```python
from build123d import *

# Parameters (mm, degrees)
F0_W     = 40
F0_H     = 3
F1_DEPTH = 12.5
F2_DEPTH = 9.5
F0_R     = 3.73
F3_DEPTH = 9.5
F4_DEPTH = 1.5
F5_W     = 13
F5_H     = 3
F6_DEPTH = 40


with BuildPart() as f1:
    # F0 (on Right) → F1 (new body, symmetric)
    with BuildSketch(Plane.YZ):
        with Locations((20, 1.5)):
            Rectangle(F0_W, F0_H)
    extrude(amount=F1_DEPTH, both=True)

    # F0 (on Right) → F2 (join, symmetric)
    with BuildSketch(Plane.YZ):
        Polygon((0, 7), (0, 3), (40, 3), (40, 7), (28.54, 7), align=None)
    extrude(amount=F2_DEPTH, both=True)

    # F0 (on Right) → F3 (join, symmetric)
    with BuildSketch(Plane.YZ):
        with BuildLine():
            Line((28.54, 7), (40, 7))
            Line((40, 7), (40, 18.87))
            ThreePointArc((40, 18.87), (37.212814, 23.786579), (31.562741, 23.920114))
            ThreePointArc((31.562741, 23.920114), (29.353421, 21.812814), (28.54, 18.87))
            Line((28.54, 18.87), (28.54, 7))
        make_face()
        with Locations((34.27, 18.87)):
            Circle(F0_R, mode=Mode.SUBTRACT)
    extrude(amount=F3_DEPTH, both=True)

    # F0 (on Right) → F4 (join, symmetric)
    with BuildSketch(Plane.YZ):
        with BuildLine():
            Line((31.562741, 23.920114), (0, 7))
            Line((0, 7), (28.54, 7))
            Line((28.54, 7), (28.54, 18.87))
            ThreePointArc((28.54, 18.87), (29.353421, 21.812814), (31.562741, 23.920114))
        make_face()
    extrude(amount=F4_DEPTH, both=True)

    # F5 (on face) → F6 (cut, through all)
    with BuildSketch(Plane.XZ):
        with Locations((0, 1.5)):
            Rectangle(F5_W, F5_H)
    extrude(amount=-F6_DEPTH, mode=Mode.SUBTRACT)


solid = f1.part
```
Check sheet for the modelled part. Datum: model origin and axes. Units: mm. A direction names the side the tool comes from. Round coordinates to 2 decimals unless told otherwise and drop trailing zeros. Loops run counter-clockwise (first coordinate to the right, second up) from the corner with the lowest first, then second, coordinate; pieces in that order, holes last. Notation, with made-up numbers: (46.25, 9.25) - (56.25, 9.25) arc R11 cw to (56.25, 28.25) - close; hole circle Ø11 at (32.25, -14.75). An arc over 180 degrees is marked (long way). Write item = value, one per line. Start each with the question number.
Q1. Section check D-D (y = 12.5). Record the boundary of the cut face in (x, z).
Q2. Section check C-C (z = 19.75). Record the boundary of the cut face in (x, y), plus the area to 3 significant figures.
Q3. Thickness scan on L1, parallel to Z at x = -4, y = 34.27; L2, parallel to X at y = 27.5, z = 2; L3, parallel to X at y = 13, z = 5.75. Record the ranges inside material, lowest first.
Q4. Section check A-A (y = 34.27). Record the boundary of the cut face in (x, z).
Q5. Access from +Z, -Z, +X, -X, +Y, -Y to the whole of each face (thin tool, end or side, straight path). Record for faces 1 (the face through (11, 20, 3)), 2 (the face through (6, 14, 7)), 3 (the face through (0, 20, 3)).
Q6. Release check for a two-part mould opening along X. For faces 4 (the face through (-9.5, 29, 9)), 5 (the face through (-5, 14, 7)), 6 (the face through (-6.5, 20, 1)) record: pulls with the +X half, pulls with the -X half, needs draft (parallel to the pull), parting line crosses it, or undercut.
Q7. Section check B-B (x = -2.5). Record the boundary of the cut face in (y, z), plus the area to 3 significant figures.
Q8. Depth check by flat-ended pin: P1, Ø6.5, axis at x = -6, y = 13.5, coming from the +Z side; P2, Ø6.5, axis at x = -5, z = 10.5, coming from the -Y side; P3, Ø8, axis at x = 6.5, y = 21.5, coming from the -Z side; P4, Ø1.5, axis at x = 10.5, y = 20.5, coming from the +Z side. Enter the tip coordinate at first touch or a pass-through.
Derived:
q1.outline = (-12.5, 0) - (-6.5, 0) - (-6.5, 3) - (6.5, 3) - (6.5, 0) - (12.5, 0) - (12.5, 3) - (9.5, 3) - (9.5, 7) - (1.5, 7) - (1.5, 13.7) - (-1.5, 13.7) - (-1.5, 7) - (-9.5, 7) - (-9.5, 3) - (-12.5, 3) - close
q2.outline = (-9.5, 28.61) - (-1.5, 28.61) - (-1.5, 23.78) - (1.5, 23.78) - (1.5, 28.61) - (9.5, 28.61) - (9.5, 30.65) - (-9.5, 30.65) - close; (-9.5, 37.89) - (9.5, 37.89) - (9.5, 39.93) - (-9.5, 39.93) - close
q2.area = 91.9 mm^2
q3.L1 = 3 to 15.14, 22.6 to 24.6
q3.L2 = -12.5 to -6.5, 6.5 to 12.5
q3.L3 = -9.5 to 9.5
q4.outline = (-12.5, 0) - (-6.5, 0) - (-6.5, 3) - (6.5, 3) - (6.5, 0) - (12.5, 0) - (12.5, 3) - (9.5, 3) - (9.5, 15.14) - (-9.5, 15.14) - (-9.5, 3) - (-12.5, 3) - close; (-9.5, 22.6) - (9.5, 22.6) - (9.5, 24.6) - (-9.5, 24.6) - close
q5.face_1 = +Z, +X, +Y, -Y
q5.face_2 = +Z, +X, -Y
q5.face_3 = -Z, +Y, -Y
q6.face_4 = pulls with the -X half
q6.face_5 = needs draft
q6.face_6 = undercut
q7.outline = (0, 3) - (40, 3) - (40, 18.87) arc R5.73 ccw to (28.54, 18.87) - (28.54, 7) - (0, 7) - close; hole circle Ø7.46 at (34.27, 18.87)
q7.area = 304 mm^2
q8.P1 = 7
q8.P2 = 28.54
q8.P3 = 0
q8.P4 = 3
